```python
from build123d import *

# Parameters (mm, degrees)
SKETCH1_W               = 100
SKETCH1_H               = 35
BOSS_EXTRUDE1_DEPTH     = 10
CUT_EXTRUDE1_DEPTH      = 54.909646632
CHAMFER1_SIZE           = 10
CHAMFER1_SIZE2          = 7.812856265
SKETCH3_W               = 2
SKETCH3_H               = 8
BOSS_EXTRUDE2_DEPTH     = 40
FILLET1_R               = 4
SKETCH4_R               = 1.75
CUT_EXTRUDE2_DEPTH      = 81.942510463
LPATTERN1_COUNT         = 7
LPATTERN1_PITCH         = 5
MIRROR1_COPY_1_SKETCH_R = 1.75
MIRROR1_COPY_1_DEPTH    = 81.942510463
MIRROR1_COPY_2_SKETCH_R = 1.75
MIRROR1_COPY_2_DEPTH    = 81.942510463
MIRROR1_COPY_3_SKETCH_R = 1.75
MIRROR1_COPY_3_DEPTH    = 81.942510463
MIRROR1_COPY_4_SKETCH_R = 1.75
MIRROR1_COPY_4_DEPTH    = 81.942510463
MIRROR1_COPY_5_SKETCH_R = 1.75
MIRROR1_COPY_5_DEPTH    = 81.942510463
MIRROR1_COPY_6_SKETCH_R = 1.75
MIRROR1_COPY_6_DEPTH    = 81.942510463
FILLET1_OF_MIRROR1_R    = 4
FILLET2_R               = 4


with BuildPart() as part:
    # Sketch1 → Boss-Extrude1 (new body)
    with BuildSketch(Plane(origin=(0, 0, 0), x_dir=(1, 0, 0), z_dir=(0, 1, 0))):
        Rectangle(SKETCH1_W, SKETCH1_H)
    extrude(amount=BOSS_EXTRUDE1_DEPTH)

    # Sketch2 → Cut-Extrude1 (cut, through all)
    with BuildSketch(Plane(origin=(0, 10, 0), x_dir=(1, 0, 0), z_dir=(0, 1, 0))):
        Polygon((-50, 17.5), (-35, 17.5), (-50, -17.5), align=None)
        Polygon((50, 17.5), (35, 17.5), (50, -17.5), align=None)
    extrude(amount=-CUT_EXTRUDE1_DEPTH, mode=Mode.SUBTRACT)

    # Chamfer1
    chamfer1_edges = [part.edges().sort_by_distance(p)[0] for p in [
        (0, 10, -17.5),
        (-42.5, 10, 0),
        (42.5, 10, 0),
    ]]
    chamfer1_side = [part.faces().sort_by_distance(p)[0] for p in [
        (0, 10, 1.029411765),
    ]]
    chamfer(chamfer1_edges, length=CHAMFER1_SIZE, length2=CHAMFER1_SIZE2, reference=chamfer1_side[0])

    # Sketch3 → Boss-Extrude2 (add)
    with BuildSketch(Plane(origin=(0, 10, 0), x_dir=(1, 0, 0), z_dir=(0, 1, 0))):
        with Locations((-10.2, -13.5)):
            Rectangle(SKETCH3_W, SKETCH3_H)
    boss_extrude2 = extrude(amount=BOSS_EXTRUDE2_DEPTH)

    # Fillet1
    fillet1_edges = [part.edges().sort_by_distance(p)[0] for p in [
        (-10.2, 50, 9.5),
        (-10.2, 50, 17.5),
    ]]
    fillet(fillet1_edges, radius=FILLET1_R - 0.0001)  # a hair under: the kernel refuses the full size

    # Sketch4 → Cut-Extrude2 (cut, through all)
    with BuildSketch(Plane.ZY.offset(11.2)):
        with Locations((13.5, 46)):
            Circle(SKETCH4_R)
    cut_extrude2 = extrude(amount=-CUT_EXTRUDE2_DEPTH, mode=Mode.SUBTRACT)

    # LPattern1: Cut-Extrude2 ×7
    with Locations(*[(0, -i * LPATTERN1_PITCH, 0) for i in range(1, LPATTERN1_COUNT)]):
        add(cut_extrude2, mode=Mode.SUBTRACT)

    # Mirror1: Boss-Extrude2, Cut-Extrude2 across plane
    add(boss_extrude2.mirror(Plane(origin=(0, 0, 0), x_dir=(0, 0, 1), z_dir=(1, 0, 0))))
    add(cut_extrude2.mirror(Plane(origin=(0, 0, 0), x_dir=(0, 0, 1), z_dir=(1, 0, 0))), mode=Mode.SUBTRACT)

    # Mirror1 copy 1 sketch → Mirror1 copy 1 (cut, through all)
    with BuildSketch(Plane(origin=(11.2, -5, 0), x_dir=(0, 0, 1), z_dir=(1, 0, 0))):
        with Locations((13.5, -46)):
            Circle(MIRROR1_COPY_1_SKETCH_R)
    extrude(amount=-MIRROR1_COPY_1_DEPTH, mode=Mode.SUBTRACT)

    # Mirror1 copy 2 sketch → Mirror1 copy 2 (cut, through all)
    with BuildSketch(Plane(origin=(11.2, -10, 0), x_dir=(0, 0, 1), z_dir=(1, 0, 0))):
        with Locations((13.5, -46)):
            Circle(MIRROR1_COPY_2_SKETCH_R)
    extrude(amount=-MIRROR1_COPY_2_DEPTH, mode=Mode.SUBTRACT)

    # Mirror1 copy 3 sketch → Mirror1 copy 3 (cut, through all)
    with BuildSketch(Plane(origin=(11.2, -15, 0), x_dir=(0, 0, 1), z_dir=(1, 0, 0))):
        with Locations((13.5, -46)):
            Circle(MIRROR1_COPY_3_SKETCH_R)
    extrude(amount=-MIRROR1_COPY_3_DEPTH, mode=Mode.SUBTRACT)

    # Mirror1 copy 4 sketch → Mirror1 copy 4 (cut, through all)
    with BuildSketch(Plane(origin=(11.2, -20, 0), x_dir=(0, 0, 1), z_dir=(1, 0, 0))):
        with Locations((13.5, -46)):
            Circle(MIRROR1_COPY_4_SKETCH_R)
    extrude(amount=-MIRROR1_COPY_4_DEPTH, mode=Mode.SUBTRACT)

    # Mirror1 copy 5 sketch → Mirror1 copy 5 (cut, through all)
    with BuildSketch(Plane(origin=(11.2, -25, 0), x_dir=(0, 0, 1), z_dir=(1, 0, 0))):
        with Locations((13.5, -46)):
            Circle(MIRROR1_COPY_5_SKETCH_R)
    extrude(amount=-MIRROR1_COPY_5_DEPTH, mode=Mode.SUBTRACT)

    # Mirror1 copy 6 sketch → Mirror1 copy 6 (cut, through all)
    with BuildSketch(Plane(origin=(11.2, -30, 0), x_dir=(0, 0, 1), z_dir=(1, 0, 0))):
        with Locations((13.5, -46)):
            Circle(MIRROR1_COPY_6_SKETCH_R)
    extrude(amount=-MIRROR1_COPY_6_DEPTH, mode=Mode.SUBTRACT)

    # Fillet1 of Mirror1
    fillet1_of_mirror1_edges = [part.edges().sort_by_distance(p)[0] for p in [
        (10.2, 50, 9.5),
        (10.2, 50, 17.5),
    ]]
    fillet(fillet1_of_mirror1_edges, radius=FILLET1_OF_MIRROR1_R - 0.0001)  # a hair under: the kernel refuses the full size

    # Fillet2
    fillet2_edges = [part.edges().sort_by_distance(p)[0] for p in [
        (9.2, 10, 13.5),
        (10.2, 10, 9.5),
        (11.2, 10, 13.5),
        (-9.2, 10, 13.5),
        (-10.2, 10, 9.5),
        (-11.2, 10, 13.5),
    ]]
    fillet(fillet2_edges, radius=FILLET2_R)


solid = part.part
```
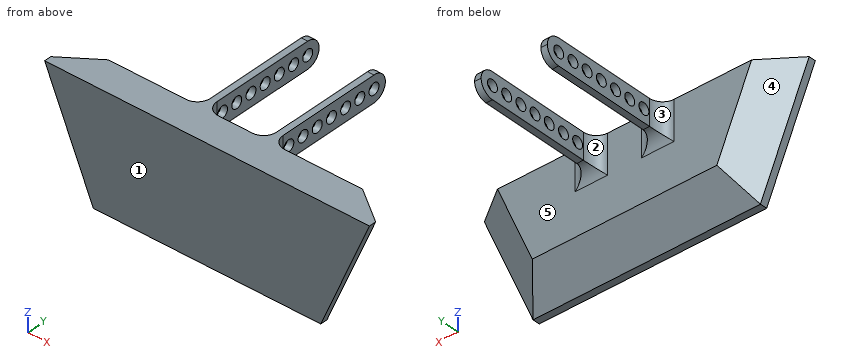
The model under review builds one solid part; all positions refer to its coordinate system, in mm. Face numbers are marked on the shaded views. A direction names the side the tool comes from. Give positions to 0.01 mm unless a question says otherwise; leave off trailing zeros. Write each loop counter-clockwise with the first axis right and the second up, starting at its lowest first coordinate (ties: lowest second). Pieces come first, ordered by that corner, then holes. Notation, with made-up numbers: M -29.75,-22 L -15.75,-22 A33 ccw -15.75,12 Z; hole C 32,3.5 d1. An arc over 180 degrees is marked long. Write each question's results on one line, items separated by ' | '. Start each with the question number.
1. We need section D-D (z = -4.5). Write out the cut boundary in (x, y).
2. For the marked faces 4 and 5, list the 3-axis set-ups (+Z, -Z, +X, -X, +Y, -Y) from which the entire face can be reached by the end or side of a thin tool; tool diameter is ignored.
3. We need section B-B (y = 11.5). Write out the cut boundary in (x, z), and give its area (3 significant figures).
4. Insertion check: pin 1 Ø5.5 at (y, z) = (46, 13.5) entering from +X; pin 2 Ø1 at (x, z) = (-24, 3.5) entering from +Y; pin 3 Ø0.6 at (x, y) = (10, 35) entering from -Z. Each pin has a flat end and moves straight along its axis. Give the tip position at first contact, or say it passes through.
5. Mouldability with a two-part tool opening along X and no side actions: class the marked faces 1, 2 and 3 as released by +X, released by -X, zero draft, split by the parting line, or undercut.
6. We need section A-A (y = 31). Write out the cut boundary in (x, z), and give its area (3 significant figures).
7. For probe 1 along Y at (x, z) = (-17.5, 12.5); probe 2 along Z at (x, y) = (10, 36); probe 3 along X at (y, z) = (5, 9), list the stretches that pass through material, from the lowest coordinate up. Write a range as [from, to].
8. We need section C-C (x = -3.5). Write out the cut boundary in (y, z).
Results found:
1) outline: M -40.57,0 L 40.57,0 L 40.57,2.19 L 29.69,10 L -29.69,10 L -40.57,2.19 Z
2) face 4: -Z, -X, +Y | face 5: -Z, +Y
3) outline: M -12.08,8.62 L -8.32,8.62 L -8.32,17.5 L -12.08,17.5 Z; M 8.32,8.62 L 12.08,8.62 L 12.08,17.5 L 8.32,17.5 Z | area: 66.7 mm^2
4) pin 1: stops at x = 11.2 | pin 2: stops at y = 10 | pin 3: stops at z = 9.5
5) face 1: zero draft | face 2: undercut | face 3: released by -X
6) outline: M -11.2,9.5 L -9.2,9.5 L -9.2,11.75 L -11.2,11.75 Z; M -11.2,15.25 L -9.2,15.25 L -9.2,17.5 L -11.2,17.5 Z; M 9.2,9.5 L 11.2,9.5 L 11.2,11.75 L 9.2,11.75 Z; M 9.2,15.25 L 11.2,15.25 L 11.2,17.5 L 9.2,17.5 Z | area: 18.0 mm^2
7) probe 1: y = [0, 10] | probe 2: z = [9.5, 11.75], [15.25, 17.5] | probe 3: x = [-42.44, 42.44]
8) outline: M 0,-17.5 L 2.19,-17.5 L 10,-7.5 L 10,17.5 L 0,17.5 Z
